Part print with two shaded views. Sizes in mm from the minimum x, y, z corner. Round coordinates to 2 decimals unless told otherwise and drop trailing zeros. Loops run counter-clockwise (first coordinate to the right, second up) from the corner with the lowest first, then second, coordinate; pieces in that order, holes last. Notation, with made-up numbers: (33, 74.5) - (49, 74.5) arc R31 ccw to (49, 103.5) - close; hole circle Ø10 at (50.5, 11). An arc over 180 degrees is marked (long way). Put each result on its own line as item: value. Start each with the question number.
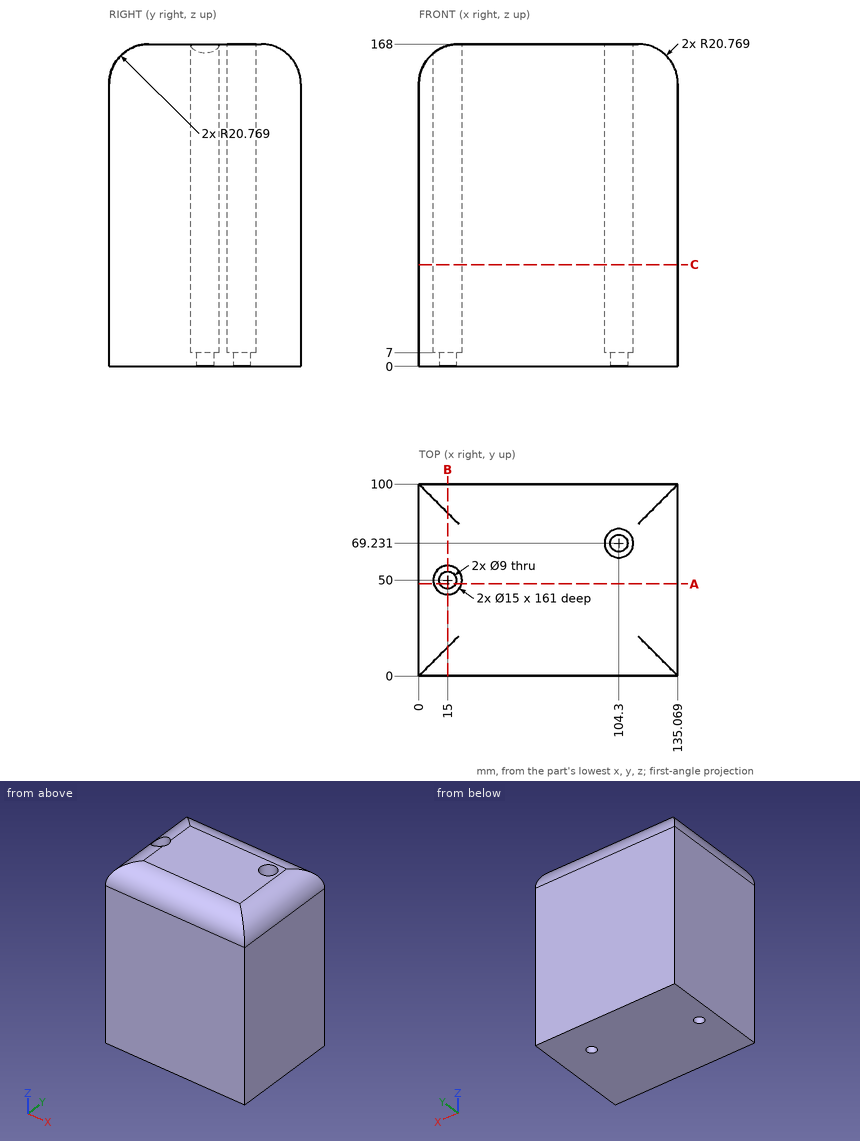
1) Drop a flat-ended pin along its axis: pin 1 Ø4.5 at (x, y) = (107, 71.5) entering from +Z. Give the stop position or say it passes through.
2) Drill centre lines: line 1 (X direction, y = 66.5, z = 119) (1 decimal); line 2 (X direction, y = 43.5, z = 114) (1 decimal); line 3 (Z direction, x = 115.5, y = 78) (1 decimal). Where is each one in solid material? Low to high. Write a range as [from, to].
3) Slice it at B-B, the plane x = 15. Write the cut outline in (y, z).
4) Slice it at A-A, the plane y = 48. Write the cut outline in (x, z).
5) Slice it at C-C, the plane z = 53. Write the cut outline in (x, y).
Taken from the geometry:
1. pin 1: stops at z = 7
2. line 1: x = [0, 97.3], [111.3, 135.1]
2. line 2: x = [0, 11.3], [18.7, 135.1]
2. line 3: z = [0, 168]
3. outline: (0, 0) - (45.5, 0) - (45.5, 7) - (42.5, 7) - (42.5, 167.18) - (15, 167.18) arc R20.77 ccw to (0, 147.23) - close; (54.5, 0) - (100, 0) - (100, 147.23) arc R20.77 ccw to (85, 167.18) - (57.5, 167.18) - (57.5, 7) - (54.5, 7) - close
4. outline: (0, 0) - (10.97, 0) - (10.97, 7) - (7.77, 7) - (7.77, 163.43) arc R20.77 ccw to (0, 147.23) - close; (19.03, 0) - (135.07, 0) - (135.07, 147.23) arc R20.77 ccw to (114.3, 168) - (22.23, 168) - (22.23, 7) - (19.03, 7) - close
5. outline: (0, 0) - (135.07, 0) - (135.07, 100) - (0, 100) - close; hole circle Ø15 at (15, 50); hole circle Ø15 at (104.3, 69.23)
